Input: part model. Units: mm. Frame: model coordinates. A direction names the side the tool comes from. Round coordinates to 2 decimals unless told otherwise and drop trailing zeros. Write each loop counter-clockwise with the first axis right and the second up, starting at its lowest first coordinate (ties: lowest second). Pieces come first, ordered by that corner, then holes. Notation, with made-up numbers: (-38, 84) -> (11, 84) arc R14 cw to (11, 105) -> close; hole circle Ø9 at (16, -21.5). An arc over 180 degrees is marked (long way). Use CSV: the item, a comma, the result in double quotes.
Autodesk Inventor part; units mm, degrees
ref_plane "Work Plane1" through (0, 0, 0) normal (-1, 0, 0) x (0, 0, 1)
ref_plane "Work Plane3" through (320, 0, 0) normal (-1, 0, 0) x (0, 0, 1)
ref_plane "YZ Plane" through (0, 0, 0) normal (1, 0, 0) x (0, 1, 0)
sketch "Sketch1" plane through (0, 0, 0) normal (1, 0, 0) x (0, 1, 0)
  circle A0 centre (0, 0) radius 200
extrude "Extrusion1" add sketch "Sketch1" along normal blind 370
sketch "Sketch2" plane through (0, 0, 0) normal (-1, 0, 0) x (0, 0, 1)
  point P0 (0, 0)
sketch "Sketch3" plane through (370, 0, 0) normal (1, 0, 0) x (0, 0, -1)
  circle A0 centre (0, 0) radius 195
  dimension "d2" = 390
extrude "Extrusion2" cut sketch "Sketch3" against normal blind 370
ref_plane "Work Plane1" through (0, 0, 0) normal (-1, 0, 0) x (0, 0, 1)
sketch "Sketch4" plane through (0, 0, 0) normal (-1, 0, 0) x (0, 0, 1)
  point P0 (0, 0)
sketch "Sketch5" plane through (0, 0, 0) normal (-1, 0, 0) x (0, 0, 1)
  line L0 (240, -99.4113) -> (99.4113, -240)
  line L1 (99.4113, -240) -> (-99.4113, -240)
  line L2 (-99.4113, -240) -> (-240, -99.4113)
  line L3 (-240, -99.4113) -> (-240, 99.4113)
  line L4 (-240, 99.4113) -> (-99.4113, 240)
  line L5 (-99.4113, 240) -> (99.4113, 240)
  line L6 (99.4113, 240) -> (240, 99.4113)
  line L7 (240, 99.4113) -> (240, -99.4113)
  point P0 (0, 0)
  point P1 (0, 0)
extrude "BackPlate" add sketch "Sketch5" along normal blind 8
fillet "Fillet1" radius 20 8 edges at (-4, -240, 99.4113) (-4, -240, -99.4113) (-4, -99.4113, -240) (-4, 99.4113, -240) (-4, 240, -99.4113) (-4, 240, 99.4113) (-4, 99.4113, 240) (-4, -99.4113, 240)
ref_plane "Work Plane3" through (320, 0, 0) normal (-1, 0, 0) x (0, 0, 1)
sketch "Sketch6" plane through (320, 0, 0) normal (-1, 0, 0) x (0, 0, 1)
  line L0 (91.127, 240) -> (-91.127, 240)
  line L1 (99.4113, 240) -> (240, 99.4113)
  line L2 (240, 99.4113) -> (240, -99.4113)
  line L3 (240, -99.4113) -> (99.4113, -240)
  line L4 (99.4113, -240) -> (-99.4113, -240)
  line L5 (-99.4113, -240) -> (-240, -99.4113)
  line L6 (-240, -99.4113) -> (-240, 99.4113)
  line L7 (-240, 99.4113) -> (-99.4113, 240)
  line L8 (-99.4113, 240) -> (99.4113, 240)
  point P0 (0, 0)
  point P1 (0, 0)
  point P2 (0, 240)
extrude "FrontPlate" add sketch "Sketch6" along normal blind 8
sketch "Sketch7" plane through (320, 0, 0) normal (1, 0, 0) x (0, 0, -1)
  circle A0 centre (0, 0) radius 195
extrude "Extrusion5" cut sketch "Sketch7" against normal blind 8
fillet "Fillet2" radius 20 8 edges at (316, -99.4113, 240) (316, 99.4113, 240) (316, 240, 99.4113) (316, 240, -99.4113) (316, 99.4113, -240) (316, -99.4113, -240) (316, -240, -99.4113) (316, -240, 99.4113)
sketch "BackplateHoles" plane through (0, 0, 0) normal (1, 0, 0) x (0, 0, -1)
  circle A0 centre (-88, 212) radius 18
  circle A1 centre (-88, -212) radius 18
  circle A2 centre (-212, 88) radius 18
  circle A3 centre (-212, -88) radius 18
  circle A4 centre (-190, 122) radius 10
  circle A5 centre (-122, 190) radius 10
  circle A6 centre (-144, 176) radius 8
  circle A7 centre (-176, 144) radius 8
  circle A8 centre (-162, 162) radius 6
  line L0 (-240, 0) -> (240, 0) construction
  circle A9 centre (-190, -122) radius 10
  circle A10 centre (-176, -144) radius 8
  circle A11 centre (-162, -162) radius 6
  circle A12 centre (-144, -176) radius 8
  circle A13 centre (-122, -190) radius 10
  circle A14 centre (88, 212) radius 18
  circle A15 centre (212, 88) radius 18
  circle A16 centre (190, 122) radius 10
  circle A17 centre (122, 190) radius 10
  circle A18 centre (144, 176) radius 8
  circle A19 centre (176, 144) radius 8
  circle A20 centre (162, 162) radius 6
  circle A21 centre (88, -212) radius 18
  circle A22 centre (212, -88) radius 18
  circle A23 centre (190, -122) radius 10
  circle A24 centre (162, -162) radius 6
  circle A25 centre (144, -176) radius 8
  circle A26 centre (122, -190) radius 10
  circle A27 centre (176, -144) radius 8
  point P0 (0, 0)
  point P1 (0, 0)
sketch "FrontplateHoles" plane through (320, 0, 0) normal (1, 0, 0) x (0, 0, -1)
  circle A0 centre (-88, 212) radius 18
  circle A1 centre (-88, -212) radius 18
  circle A2 centre (-212, 88) radius 18
  circle A3 centre (-212, -88) radius 18
  circle A4 centre (-190, 122) radius 10
  circle A5 centre (-122, 190) radius 10
  circle A6 centre (-144, 176) radius 8
  circle A7 centre (-176, 144) radius 8
  circle A8 centre (-162, 162) radius 6
  circle A9 centre (50, -222) radius 10
  circle A10 centre (24, -226) radius 8
  circle A11 centre (0, -228) radius 6
  circle A12 centre (-24, -226) radius 8
  circle A13 centre (-50, -222) radius 10
  circle A14 centre (-190, -122) radius 10
  circle A15 centre (-176, -144) radius 8
  circle A16 centre (-162, -162) radius 6
  circle A17 centre (-144, -176) radius 8
  circle A18 centre (-122, -190) radius 10
  circle A19 centre (88, 212) radius 18
  circle A20 centre (212, 88) radius 18
  circle A21 centre (190, 122) radius 10
  circle A22 centre (122, 190) radius 10
  circle A23 centre (144, 176) radius 8
  circle A24 centre (176, 144) radius 8
  circle A25 centre (162, 162) radius 6
  circle A26 centre (88, -212) radius 18
  circle A27 centre (212, -88) radius 18
  circle A28 centre (190, -122) radius 10
  circle A29 centre (162, -162) radius 6
  circle A30 centre (144, -176) radius 8
  circle A31 centre (122, -190) radius 10
  circle A32 centre (176, -144) radius 8
  circle A33 centre (222.0138, -50) radius 10
  circle A34 centre (226, -24) radius 8
  circle A35 centre (228.0138, 0) radius 6
  circle A36 centre (226, 24) radius 8
  circle A37 centre (222.0138, 50) radius 10
  circle A38 centre (-222, -50) radius 10
  circle A39 centre (-226, -24) radius 8
  circle A40 centre (-228, 0) radius 6
  circle A41 centre (-226, 24) radius 8
  circle A42 centre (-222, 50) radius 10
  circle A43 centre (50, 222) radius 10
  circle A44 centre (24, 226) radius 8
  circle A45 centre (0, 228) radius 6
  circle A46 centre (-24, 226) radius 8
  circle A47 centre (-50, 222) radius 10
  point P0 (0, 0)
  point P1 (0, 0)
hole "Hole1" at (0, -212, -88) at (0, -88, -212) at (0, 88, -212) at (0, 212, -88) at (0, 212, 88) at (0, 88, 212) at (0, -88, 212) at (0, -212, 88) direction (-1, 0, 0) diameter 36 depth 8
hole "Hole2" at (0, -190, 122) at (0, -122, 190) at (0, 122, 190) at (0, 190, 122) at (0, 190, -122) at (0, 122, -190) at (0, -122, -190) at (0, -190, -122) direction (-1, 0, 0) diameter 20 depth 8
hole "Hole3" at (0, -144, 176) at (0, 176, 144) at (0, 144, 176) at (0, -176, 144) at (0, -176, -144) at (0, -144, -176) at (0, 144, -176) at (0, 176, -144) direction (-1, 0, 0) diameter 16 depth 8
hole "Hole4" at (0, -162, 162) at (0, 162, 162) at (0, 162, -162) at (0, -162, -162) direction (-1, 0, 0) diameter 12 depth 8
hole "Hole5" at (320, -88, 212) at (320, 88, 212) at (320, 212, 88) at (320, 212, -88) at (320, -212, -88) at (320, -212, 88) at (320, -88, -212) at (320, 88, -212) direction (-1, 0, 0) diameter 36 depth 8
hole "Hole6" at (320, 222, 50) at (320, 222, -50) at (320, -222, 50) at (320, -222, -50) direction (-1, 0, 0) diameter 20 depth 8
hole "Hole7" at (320, -226, 24) at (320, -226, -24) at (320, 226, -24) at (320, 226, 24) direction (-1, 0, 0) diameter 16 depth 8
hole "Hole8" at (320, 228, 0) at (320, -228, 0) direction (-1, 0, 0) diameter 12 depth 8
properties part number "Primary"
Item 1: First-contact query: pin 1 Ø1 at (x, z) = (143, 83.5) entering from +Y; pin 2 Ø18.5 at (y, z) = (226, -24) entering from +X; pin 3 Ø13 at (y, z) = (226, 24) entering from +X. Flat tips, straight axial feed; report the tip coordinate or a pass-through.
Worked answers:
pin 1,"stops at y = 181.96"
pin 2,"stops at x = 320"
pin 3,"stops at x = 0"
Item 2: Section query D-D on x = 282.5. Return the cut outline in (y, z).
Worked answers:
outline,"circle Ø400 at (0, 0); hole circle Ø390 at (0, 0)"
Item 3: Pull-direction query (Z, two-part tool) for faces 1 (the face through (370, 192, -44)), 2 (the face through (-4.06, 113.57, 184.62)), 3 (the face through (315.944, 72.822, -221.677)), 4 (the face through (-3.94, -170.61, -168.8)); classes: +Z half, -Z half, draft (parallel to the pull), parting line (faces both ways), or undercut.
Worked answers:
face 1,"draft"
face 2,"undercut"
face 3,"undercut"
face 4,"-Z half"
Item 4: Section query C-C on z = -211. Return the cut outline in (x, y).
Worked answers:
outline,"(-8, -128.41) -> (0, -128.41) -> (0, -105.97) -> (-8, -105.97) -> close; (-8, -70.03) -> (0, -70.03) -> (0, 70.03) -> (-8, 70.03) -> close; (-8, 105.97) -> (0, 105.97) -> (0, 128.41) -> (-8, 128.41) -> close; (312, -128.41) -> (320, -128.41) -> (320, -105.97) -> (312, -105.97) -> close; (312, -70.03) -> (320, -70.03) -> (320, 70.03) -> (312, 70.03) -> close; (312, 105.97) -> (320, 105.97) -> (320, 128.41) -> (312, 128.41) -> close"
Item 5: Line query: line 1 (Y direction, x = -4, z = -88); line 2 (X direction, y = -45, z = 199.5); line 3 (Z direction, x = -4, y = 144). Output: solid intervals per line, ascending.
Worked answers:
line 1,"y = -240 to -230, -194 to 194, 230 to 240"
line 2,"x = -8 to 0, 312 to 320"
line 3,"z = -195.41 to -184, -168 to 168, 184 to 195.41"
Item 6: Set-up query: faces 5 (the face through (316, 222, 60)), 6 (the face through (-4.06, -136.19, -174.27)), 7 (the face through (316.06, -168.8, 170.61)). Return all of +Z, -Z, +X, -X, +Y, -Y with unobstructed straight access to the full face (end or side cutting, diameter ignored); none if empty.
Worked answers:
face 5,"+X"
face 6,"-X"
face 7,"+Z, +X, -X, -Y"
Item 7: Section query B-B on y = 144. Return the cut outline in (x, z).
Worked answers:
outline,"(-8, -195.41) -> (0, -195.41) -> (0, -184) -> (-8, -184) -> close; (-8, -168) -> (0, -168) -> (0, -138.79) -> (312, -138.79) -> (312, -195.41) -> (320, -195.41) -> (320, -138.79) -> (370, -138.79) -> (370, -131.49) -> (0, -131.49) -> (0, 131.49) -> (370, 131.49) -> (370, 138.79) -> (320, 138.79) -> (320, 195.41) -> (312, 195.41) -> (312, 138.79) -> (0, 138.79) -> (0, 168) -> (-8, 168) -> close; (-8, 184) -> (0, 184) -> (0, 195.41) -> (-8, 195.41) -> close"
Item 8: Section query A-A on z = 122. Return the cut outline in (x, y).
Worked answers:
outline,"(-8, -217.41) -> (0, -217.41) -> (0, -200) -> (-8, -200) -> close; (-8, -180) -> (0, -180) -> (0, -158.48) -> (312, -158.48) -> (312, -217.41) -> (320, -217.41) -> (320, -158.48) -> (370, -158.48) -> (370, -152.12) -> (0, -152.12) -> (0, 152.12) -> (370, 152.12) -> (370, 158.48) -> (320, 158.48) -> (320, 217.41) -> (312, 217.41) -> (312, 158.48) -> (0, 158.48) -> (0, 180) -> (-8, 180) -> close; (-8, 200) -> (0, 200) -> (0, 217.41) -> (-8, 217.41) -> close"
